from build123d import *

# Parameters (mm, degrees)
SKETCH1_W                      = 65
SKETCH1_H                      = 100
BOSS_EXTRUDE1_DEPTH            = 5
SKETCH2_R                      = 3
BOSS_EXTRUDE2_DEPTH            = 3
F_3_6_3_6_DIAMETER_HOLE1_D     = 3.6
CBORE_FOR_M3_SHCS1_D           = 3.4
CBORE_FOR_M3_SHCS1_CBORE_D     = 6.5
CBORE_FOR_M3_SHCS1_CBORE_DEPTH = 3
SKETCH9_W                      = 100
SKETCH9_H                      = 5
BOSS_EXTRUDE3_DEPTH            = 50
CBORE_FOR_M3_SHCS2_D           = 3.4
CBORE_FOR_M3_SHCS2_CBORE_D     = 6.5
CBORE_FOR_M3_SHCS2_CBORE_DEPTH = 3
CUT_EXTRUDE1_DEPTH             = 1
FILLET1_R                      = 1
FILLET2_R                      = 5
F_5_1_5_1_DIAMETER_HOLE1_D     = 5.1


with BuildPart() as part:
    # Sketch1 → Boss-Extrude1 (new body)
    with BuildSketch(Plane(origin=(0, 0, 0), x_dir=(1, 0, 0), z_dir=(0, 1, 0))):
        with Locations((32.5, -50)):
            Rectangle(SKETCH1_W, SKETCH1_H)
    extrude(amount=BOSS_EXTRUDE1_DEPTH)

    # Sketch2 → Boss-Extrude2 (add)
    with BuildSketch(Plane(origin=(0, 5, 0), x_dir=(1, 0, 0), z_dir=(0, 1, 0))):
        with Locations(Location((8, -21, 0), (0, 0, 270))):
            Circle(SKETCH2_R)
        with Locations(Location((57, -21, 0), (0, 0, 270))):
            Circle(SKETCH2_R)
        with Locations(Location((57, -79, 0), (0, 0, 270))):
            Circle(SKETCH2_R)
        with Locations(Location((8, -79, 0), (0, 0, 270))):
            Circle(SKETCH2_R)
    extrude(amount=BOSS_EXTRUDE2_DEPTH)

    # Ø3.6 (3.6) Diameter Hole1 (through all)
    with Locations(Plane(origin=(0, 8, 0), x_dir=(1, 0, 0), z_dir=(0, 1, 0))):
        with Locations((8, -21), (57, -21), (57, -79), (8, -79)):
            Hole(F_3_6_3_6_DIAMETER_HOLE1_D / 2)

    # CBORE for M3 SHCS1 (through all)
    with Locations(Plane(origin=(0, 5, 0), x_dir=(1, 0, 0), z_dir=(0, 1, 0))):
        with Locations((13.75, -7.5), (51.25, -7.5)):
            CounterBoreHole(CBORE_FOR_M3_SHCS1_D / 2, CBORE_FOR_M3_SHCS1_CBORE_D / 2, CBORE_FOR_M3_SHCS1_CBORE_DEPTH)

    # Sketch9 → Boss-Extrude3 (add)
    with BuildSketch(Plane.ZY):
        with Locations((50, 2.5)):
            Rectangle(SKETCH9_W, SKETCH9_H)
    extrude(amount=BOSS_EXTRUDE3_DEPTH)

    # CBORE for M3 SHCS2 (through all)
    with Locations(Plane(origin=(0, 5, 0), x_dir=(1, 0, 0), z_dir=(0, 1, 0))):
        with Locations((-23.75, -67.5), (-23.75, -7.5), (-23.75, -37.5)):
            CounterBoreHole(CBORE_FOR_M3_SHCS2_D / 2, CBORE_FOR_M3_SHCS2_CBORE_D / 2, CBORE_FOR_M3_SHCS2_CBORE_DEPTH)

    # Sketch16 → Cut-Extrude1 (cut)
    with BuildSketch(Plane(origin=(0, 5, 0), x_dir=(1, 0, 0), z_dir=(0, 1, 0))):
        with BuildLine():
            Line((39.126262207, -50.847545166), (39.126262207, -49.597897606))
            add(Edge.make_bspline(
                [(39.126262207, -49.597897606), (38.887061603, -49.575713781), (38.426953933, -49.5330427), (37.765335099, -49.467029699), (37.16050318, -49.395654418), (36.608878249, -49.329176979), (36.103389832, -49.260432621), (35.637684233, -49.194155672), (35.207796553, -49.125451167), (34.693851603, -49.042468377), (34.106849427, -48.930569543), (33.65316464, -48.833024779), (33.43663372, -48.786469421)],
                knots=[0, 0, 0, 0, 1.253096053, 2.41035807, 3.468180285, 4.429891672, 5.308555075, 6.129167563, 6.883542428, 7.579384342, 8.844708592, 10, 10, 10, 10], degree=3))
            add(Edge.make_bspline(
                [(33.43663372, -48.786469421), (33.362346649, -48.767894411), (33.217288497, -48.731623541), (33.012809199, -48.653717957), (32.825678299, -48.562470211), (32.654731085, -48.453628715), (32.502165181, -48.313171441), (32.378215441, -48.129778401), (32.270782782, -47.910183348), (32.22072951, -47.746398482), (32.194209557, -47.659619598)],
                knots=[0, 0, 0, 0, 1.028706086, 2.008723763, 2.935244992, 3.824118955, 4.724963072, 5.700873389, 6.781843246, 8, 8, 8, 8], degree=3))
            add(Edge.make_bspline(
                [(32.194209557, -47.659619598), (32.184050249, -47.593155924), (32.163986257, -47.461894353), (32.185456965, -47.261992825), (32.24760698, -47.068817641), (32.345988654, -46.886281707), (32.470276431, -46.723283517), (32.612903387, -46.590894898), (32.770825068, -46.49396615), (32.885825633, -46.461994139), (32.943034973, -46.44608902)],
                knots=[0, 0, 0, 0, 1.027404461, 2.029059083, 3.048769739, 4.122307651, 5.19302046, 6.17728816, 7.093255398, 8, 8, 8, 8], degree=3))
            add(Edge.make_bspline(
                [(32.943034973, -46.44608902), (33.019790611, -46.432729059), (33.159183567, -46.408466548), (33.358775166, -46.415044291), (33.530189985, -46.45624418), (33.682659012, -46.516761006), (33.820245014, -46.588705021), (33.94106644, -46.670397622), (34.053969979, -46.753634053), (34.125488835, -46.811784665), (34.161381149, -46.840968018)],
                knots=[0, 0, 0, 0, 1.397360562, 2.537692669, 3.559369145, 4.550448304, 5.47954959, 6.34367758, 7.168761249, 8, 8, 8, 8], degree=3))
            add(Edge.make_bspline(
                [(34.161381149, -46.840968018), (34.171740761, -46.84988817), (34.20290871, -46.876725361), (34.270587507, -46.926391538), (34.365875235, -47.009106142), (34.490280901, -47.108420261), (34.623007569, -47.217425956), (34.758849499, -47.313547894), (34.885293124, -47.395630136), (35.04302611, -47.483660165), (35.248195948, -47.563686604), (35.419904702, -47.590557351), (35.50734066, -47.604240227)],
                knots=[0, 0, 0, 0, 0.26063328, 0.784141858, 1.599335041, 2.665418653, 3.819900223, 4.873162956, 5.836886495, 6.693141337, 8.316111744, 10, 10, 10, 10], degree=3))
            Line((35.50734066, -47.604240227), (39.126262207, -48.073760986))
            Line((39.126262207, -48.073760986), (39.126262207, -47.466995697))
            add(Edge.make_bspline(
                [(39.126262207, -47.466995697), (39.120615941, -47.395372643), (39.108842141, -47.246021633), (39.011762919, -47.038358034), (38.893301343, -46.84311371), (38.780591009, -46.744004371), (38.726567612, -46.696500092)],
                knots=[0, 0, 0, 0, 0.957298162, 1.996193101, 3.039551627, 4, 4, 4, 4], degree=3))
            Line((38.726567612, -46.696500092), (38.098132133, -46.282358704))
            Line((38.098132133, -46.282358704), (38.098132133, -45.608175049))
            add(Edge.make_bspline(
                [(38.098132133, -45.608175049), (38.265069197, -45.651305716), (38.590637549, -45.73542113), (39.059543061, -45.904315208), (39.510452961, -46.111726833), (39.782169404, -46.301225336), (39.9208358, -46.397933044)],
                knots=[0, 0, 0, 0, 1.033858386, 2.016278253, 2.987637474, 4, 4, 4, 4], degree=3))
            add(Edge.make_bspline(
                [(39.9208358, -46.397933044), (39.980466774, -46.441596233), (40.101066248, -46.529901979), (40.265647201, -46.68871056), (40.416093013, -46.870100588), (40.556417575, -47.068585687), (40.676744862, -47.287138148), (40.759698519, -47.527310442), (40.812591451, -47.784126696), (40.818378437, -47.961125766), (40.821352539, -48.052090797)],
                knots=[0, 0, 0, 0, 0.904302346, 1.828888262, 2.791608349, 3.786843382, 4.80268608, 5.834756118, 6.887217442, 8, 8, 8, 8], degree=3))
            Line((40.821352539, -48.052090797), (40.821352539, -54.430349731))
            Line((40.821352539, -54.430349731), (39.126262207, -54.430349731))
            Line((39.126262207, -54.430349731), (39.126262207, -52.369273987))
            add(Edge.make_bspline(
                [(39.126262207, -52.369273987), (38.824641017, -52.338588763), (38.212494456, -52.276312453), (37.278571929, -52.215269505), (36.316663871, -52.178581692), (35.66628914, -52.174105191), (35.336386948, -52.171834488)],
                knots=[0, 0, 0, 0, 0.958130554, 1.944546155, 2.957372268, 4, 4, 4, 4], degree=3))
            add(Edge.make_bspline(
                [(35.336386948, -52.171834488), (35.216918961, -52.176632011), (34.979958118, -52.18614774), (34.699390908, -52.267738632), (34.498680733, -52.345822532), (34.376377238, -52.399383952), (34.282754213, -52.45111856), (34.234840863, -52.489924695), (34.214352722, -52.506518517)],
                knots=[0, 0, 0, 0, 1.804721428, 3.579605919, 4.387653081, 5.067635593, 5.601313335, 6, 6, 6, 6], degree=3))
            add(Edge.make_bspline(
                [(34.214352722, -52.506518517), (34.158438507, -52.572803412), (34.054075473, -52.696523165), (33.974254217, -52.882970365), (33.965236632, -53.035635661), (33.99855982, -53.155268657), (34.063359986, -53.281985338), (34.125363446, -53.363077846), (34.158973351, -53.407035255)],
                knots=[0, 0, 0, 0, 1.530222605, 2.85613729, 3.495539136, 4.19786485, 5.023125643, 6, 6, 6, 6], degree=3))
            add(Edge.make_bspline(
                [(34.158973351, -53.407035255), (34.202678445, -53.453603851), (34.288209182, -53.54473845), (34.449483531, -53.638340717), (34.618180335, -53.696546772), (34.801341682, -53.734863252), (35.02056346, -53.757230953), (35.181594158, -53.781052837), (35.27378418, -53.794690857)],
                knots=[0, 0, 0, 0, 0.943448386, 1.846325613, 2.731669575, 3.584362821, 4.617048522, 6, 6, 6, 6], degree=3))
            Line((35.27378418, -53.794690857), (35.27378418, -54.543516273))
            add(Edge.make_bspline(
                [(35.27378418, -54.543516273), (35.145259799, -54.539686724), (34.899665229, -54.532368918), (34.549534649, -54.49381644), (34.23492324, -54.435411311), (33.95485327, -54.352646637), (33.704937688, -54.251951832), (33.47764334, -54.142729191), (33.274451352, -54.017945692), (33.089768771, -53.886609091), (32.927584898, -53.741089605), (32.786131125, -53.584968182), (32.654824603, -53.424803574), (32.58524624, -53.30689432), (32.550563774, -53.248120537)],
                knots=[0, 0, 0, 0, 1.463419428, 2.796417783, 4.006075808, 5.101867847, 6.114868065, 7.071137589, 7.969092879, 8.826327314, 9.648155468, 10.443549341, 11.224161887, 12, 12, 12, 12], degree=3))
            add(Edge.make_bspline(
                [(32.550563774, -53.248120537), (32.520790697, -53.193492864), (32.459254397, -53.080585998), (32.397200219, -52.890384649), (32.348206864, -52.6819503), (32.320086722, -52.457698844), (32.315640727, -52.227756787), (32.34661926, -52.004027153), (32.413206209, -51.79241002), (32.487069025, -51.66662071), (32.524077988, -51.603593979)],
                knots=[0, 0, 0, 0, 0.865492594, 1.788838003, 2.776551332, 3.847715376, 4.932865467, 5.972249091, 6.983995453, 8, 8, 8, 8], degree=3))
            add(Edge.make_bspline(
                [(32.524077988, -51.603593979), (32.599388708, -51.507318221), (32.75324726, -51.310628445), (33.055018494, -51.068656229), (33.409086865, -50.860800161), (33.672452045, -50.758731497), (33.809842529, -50.705485039)],
                knots=[0, 0, 0, 0, 0.918076197, 1.875614441, 2.891765566, 4, 4, 4, 4], degree=3))
            add(Edge.make_bspline(
                [(33.809842529, -50.705485039), (33.898631758, -50.682441773), (34.087470798, -50.633432807), (34.395240763, -50.584968257), (34.740993079, -50.551926433), (35.248657148, -50.532699083), (35.895954097, -50.531314455), (36.413618911, -50.570608952), (36.667899666, -50.589910698)],
                knots=[0, 0, 0, 0, 0.574329406, 1.22149743, 1.948877103, 2.749030755, 4.403100056, 6, 6, 6, 6], degree=3))
            Line((36.667899666, -50.589910698), (39.126262207, -50.847545166))
        make_face()
    extrude(amount=-CUT_EXTRUDE1_DEPTH, mode=Mode.SUBTRACT)

    # Fillet1
    fillet1_edges = [part.edges().sort_by_distance(p)[0] for p in [
        (8, 5, 18),
        (57, 5, 18),
        (57, 5, 76),
        (8, 5, 76),
    ]]
    fillet(fillet1_edges, radius=FILLET1_R)

    # Fillet2
    fillet2_edges = [part.edges().sort_by_distance(p)[0] for p in [
        (-50, 2.5, 0),
        (-50, 2.5, 100),
        (65, 2.5, 0),
        (65, 2.5, 100),
    ]]
    fillet(fillet2_edges, radius=FILLET2_R)

    # Ø5.1 (5.1) Diameter Hole1 (through all)
    with Locations(Plane(origin=(0, 5, 0), x_dir=(1, 0, 0), z_dir=(0, 1, 0))):
        with Locations((-38.75, -82.5), (-8.75, -52.5), (-38.75, -52.5), (-8.75, -82.5)):
            Hole(F_5_1_5_1_DIAMETER_HOLE1_D / 2)


solid = part.part
Can you work these out from the model? Positions are in its coordinate system, mm. A direction names the side the tool comes from. Coordinates: 2 decimals unless noted, no trailing zeros. Write each loop counter-clockwise with the first axis right and the second up, starting at its lowest first coordinate (ties: lowest second). Pieces come first, ordered by that corner, then holes. Notation, with made-up numbers: (-33.75, 0) - (18.25, 0) arc R32 cw to (18.25, 38) - close; hole circle Ø11 at (62, -2). An arc over 180 degrees is marked (long way). Return JSON: item names as keys, results as strings. Group by question number.
Item 1: Please list where these lines run through material, in increasing order: probe 1 along X at (y, z) = (0.65, 7.5); probe 2 along X at (y, z) = (3.5, 21); probe 3 along Z at (x, y) = (57, 3).
Item 2: If we section it at C-C (z = 67.5): Write out the boundary of the cut face in (x, y), then the cut area to 3 significant figures.
Item 3: Which directions (+Z, -Z, +X, -X, +Y, -Y) give clear straight access to the entire face, cutting with the end or side of a thin tool? Please do faces 3 (the face through (-22, 2, 69)), 4 (the face through (55, 8, 79)).
Item 4: We'd pull the mould along X, two halves only. Please class faces 1 (the face through (6, 8, 79)), 2 (the face through (12.97, 0.99, 9.01)): pulls with the +X half, pulls with the -X half, needs draft (parallel to the pull), parting line crosses it, or undercut.
Item 5: If we section it at A-A (x = -23.75): Write out the boundary of the cut face in (y, z).
Item 6: If we section it at D-D (x = -38.75): Write out the boundary of the cut face in (y, z).
Item 7: I'm going to push flat-ended pins straight in: pin 1 Ø4 at (x, z) = (-29.5, 29) entering from +Y; pin 2 Ø3 at (x, z) = (8, 79) entering from -Y; pin 3 Ø2 at (x, z) = (15.5, 8.5) entering from +Y. Where does each tip first touch, or does it pass through?
Item 8: If we section it at B-B (x = 8): Write out the boundary of the cut face in (y, z).
Return value:
{
 "1": {"probe 1": "x = -50 to -25.45, -22.05 to 12.05, 15.45 to 49.55, 52.95 to 65", "probe 2": "x = -50 to 6.2, 9.8 to 55.2, 58.8 to 65", "probe 3": "z = 0 to 19.2, 22.8 to 77.2, 80.8 to 100"},
 "2": {"outline": "(-50, 0) - (-25.45, 0) - (-25.45, 2) - (-27, 2) - (-27, 5) - (-50, 5) - close; (-22.05, 0) - (65, 0) - (65, 5) - (-20.5, 5) - (-20.5, 2) - (-22.05, 2) - close", "area": "549 mm^2"},
 "3": {"face 3": "+Y", "face 4": "+Z, -Z, +X, -X, +Y"},
 "4": {"face 1": "needs draft", "face 2": "undercut"},
 "5": {"outline": "(0, 0) - (5, 0) - (5, 4.25) - (2, 4.25) - (2, 5.8) - (0, 5.8) - close; (0, 9.2) - (2, 9.2) - (2, 10.75) - (5, 10.75) - (5, 34.25) - (2, 34.25) - (2, 35.8) - (0, 35.8) - close; (0, 39.2) - (2, 39.2) - (2, 40.75) - (5, 40.75) - (5, 64.25) - (2, 64.25) - (2, 65.8) - (0, 65.8) - close; (0, 69.2) - (2, 69.2) - (2, 70.75) - (5, 70.75) - (5, 100) - (0, 100) - close"},
 "6": {"outline": "(0, 0) - (5, 0) - (5, 49.95) - (0, 49.95) - close; (0, 55.05) - (5, 55.05) - (5, 79.95) - (0, 79.95) - close; (0, 85.05) - (5, 85.05) - (5, 100) - (0, 100) - close"},
 "7": {"pin 1": "stops at y = 5", "pin 2": "passes through", "pin 3": "stops at y = 2"},
 "8": {"outline": "(0, 0) - (5, 0) - (5, 17) arc R1 cw to (6, 18) - (8, 18) - (8, 19.2) - (0, 19.2) - close; (0, 22.8) - (8, 22.8) - (8, 24) - (6, 24) arc R1 cw to (5, 25) - (5, 75) arc R1 cw to (6, 76) - (8, 76) - (8, 77.2) - (0, 77.2) - close; (0, 80.8) - (8, 80.8) - (8, 82) - (6, 82) arc R1 cw to (5, 83) - (5, 100) - (0, 100) - close"}
}
